Can you work these out from the model? Positions are in its coordinate system, mm. Face numbers are marked on the shaded views. A direction names the side the tool comes from. Round coordinates to 2 decimals unless told otherwise and drop trailing zeros. Loops run counter-clockwise (first coordinate to the right, second up) from the corner with the lowest first, then second, coordinate; pieces in that order, holes last. Notation, with made-up numbers: (43, -12) - (99, -12) arc R31 cw to (99, 18) - close; hole circle Ø4 at (60.5, -36). An arc over 180 degrees is marked (long way). Answer as CSV lines item,"result".
```python
from build123d import *

# Parameters (mm, degrees)
SKETCH1_W           = 56
SKETCH1_H           = 48
BOSS_EXTRUDE1_DEPTH = 37
SKETCH2_R           = 21.4
CUT_EXTRUDE1_DEPTH  = 17
SKETCH4_R           = 2.5
CUT_EXTRUDE2_DEPTH  = 5


with BuildPart() as part:
    # Sketch1 → Boss-Extrude1 (new body)
    with BuildSketch(Plane.XY):
        Rectangle(SKETCH1_W, SKETCH1_H)
    extrude(amount=BOSS_EXTRUDE1_DEPTH)

    # Sketch2 → Cut-Extrude1 (cut)
    with BuildSketch(Plane.XY.offset(37)):
        Circle(SKETCH2_R)
    extrude(amount=-CUT_EXTRUDE1_DEPTH, mode=Mode.SUBTRACT)

    # Sketch4 → Cut-Extrude2 (cut)
    with BuildSketch(Plane.XZ.offset(24)):
        with Locations(Location((-24, 33.5, 0), (0, 0, 270))):
            Circle(SKETCH4_R)
        with Locations(Location((24, 33.5, 0), (0, 0, 270))):
            Circle(SKETCH4_R)
        with Locations(Location((24, 3.5, 0), (0, 0, 270))):
            Circle(SKETCH4_R)
        with Locations(Location((-24, 3.5, 0), (0, 0, 270))):
            Circle(SKETCH4_R)
    extrude(amount=-CUT_EXTRUDE2_DEPTH, mode=Mode.SUBTRACT)


solid = part.part
```
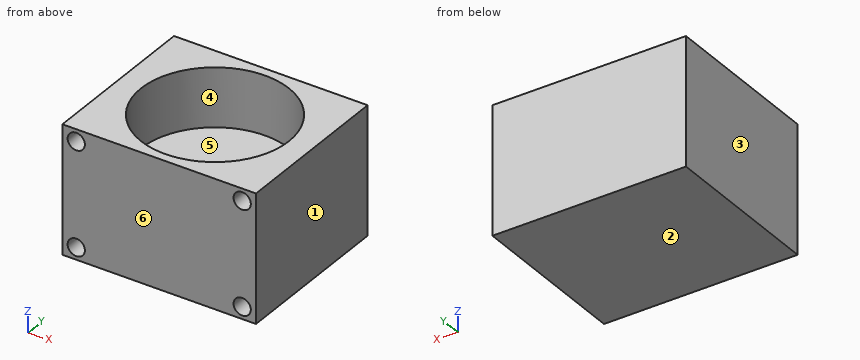
Q1. Imagine slicing it at B-B (x = -24). Write out the boundary of the cut face in (y, z), then the cut area to 3 significant figures.
Checks:
outline,"(-24, 0) - (24, 0) - (24, 37) - (-24, 37) - (-24, 36) - (-19, 36) - (-19, 31) - (-24, 31) - (-24, 6) - (-19, 6) - (-19, 1) - (-24, 1) - close"
area,"1,730 mm²"
Q2. If I drill on line 1 along Y through (x, z) = (0, 31); line 2 along X through (y, z) = (-21, 3); line 3 along Z through (x, y) = (-15.5, -4.5), over which ranges is the centre line in solid material (lowest first)? Write a range as [from, to].
Checks:
line 1,"[-24, -21.4], [21.4, 24]"
line 2,"[-28, -26.45], [-21.55, 21.55], [26.45, 28]"
line 3,"[0, 20]"
Q3. We'd pull the mould along X, two halves only. Please class the marked faces 1, 2, 3 and 4: pulls with the +X half, pulls with the -X half, needs draft (parallel to the pull), parting line crosses it, or undercut.
Checks:
face 1,"pulls with the +X half"
face 2,"needs draft"
face 3,"pulls with the -X half"
face 4,"undercut"
Q4. I'm going to push a flat-ended pin straight in: pin 1 Ø2 at (x, y) = (-3.5, -16) entering from +Z. Where does the tip first touch, or does it pass through?
Checks:
pin 1,"z = 20"
Q5. Imagine slicing it at C-C (z = 3.5). Write out the boundary of the cut face in (x, y).
Checks:
outline,"(-28, -24) - (-26.5, -24) - (-26.5, -19) - (-21.5, -19) - (-21.5, -24) - (21.5, -24) - (21.5, -19) - (26.5, -19) - (26.5, -24) - (28, -24) - (28, 24) - (-28, 24) - close"
Q6. On a 3-axis mill with a long thin cutter (end or side, diameter ignored), from which of +Z, -Z, +X, -X, +Y, -Y can I reach the whole of each face in a straight line? I mean the marked faces 5 and 6. Say none if no direction works.
Checks:
face 5,"+Z"
face 6,"+Z, -Z, +X, -X, -Y"
Q7. Imagine slicing it at A-A (z = 33.5). Write out the boundary of the cut face in (x, y), then the cut area to 3 significant figures.
Checks:
outline,"(-28, -24) - (-26.5, -24) - (-26.5, -19) - (-21.5, -19) - (-21.5, -24) - (21.5, -24) - (21.5, -19) - (26.5, -19) - (26.5, -24) - (28, -24) - (28, 24) - (-28, 24) - close; hole circle Ø42.8 at (0, 0)"
area,"1,200 mm²"
Q8. Imagine slicing it at D-D (y = 0). Write out the boundary of the cut face in (x, z), then the cut area to 3 significant figures.
Checks:
outline,"(-28, 0) - (28, 0) - (28, 37) - (21.4, 37) - (21.4, 20) - (-21.4, 20) - (-21.4, 37) - (-28, 37) - close"
area,"1,340 mm²"
